Build history of the part. All positions in model axes, mm. A direction names the side the tool comes from. Round coordinates to 2 decimals unless told otherwise and drop trailing zeros. Write each loop counter-clockwise with the first axis right and the second up, starting at its lowest first coordinate (ties: lowest second). Pieces come first, ordered by that corner, then holes. Notation, with made-up numbers: (87.5, 88.5) -> (92.5, 88.5) arc R16 cw to (92.5, 109.5) -> close; hole circle Ø5 at (11.5, 71). An arc over 180 degrees is marked (long way). Answer in a Markdown table with one row per item.
```python
from build123d import *

# Parameters (mm, degrees)
ESBO_O1_R                  = 2.5
RESSALTO_EXTRUS_O1_DEPTH   = 10.6
ESBO_O8_W                  = 21.2
ESBO_O8_H                  = 35
RESSALTO_EXTRUS_O6_DEPTH   = 1.5
RESSALTO_EXTRUS_O2_DEPTH   = 1.5
CORTE_EXTRUS_O1_DEPTH      = 48.855720661
CORTE_EXTRUS_O1_DEPTH_BACK = 48.855720661
ESBO_O3_W                  = 15.2
ESBO_O3_H                  = 37.5
CORTE_EXTRUS_O2_DEPTH      = 48.855720661
CORTE_EXTRUS_O2_DEPTH_BACK = 48.855720661
ESBO_O4_R                  = 0.85
ESBO_O5_W                  = 3
ESBO_O5_H                  = 30
RESSALTO_EXTRUS_O3_DEPTH   = 2.5
RESSALTO_EXTRUS_O4_DEPTH   = 2.5
RESSALTO_EXTRUS_O5_START   = -83.6
ESBO_O7_R                  = 35
RESSALTO_EXTRUS_O5_DEPTH   = 3
NERVURA2_REACH             = 121.79
ESBO_O10_WALL_W            = 274.68518898
ESBO_O10_WALL_H            = 2
ESBO_O11_W                 = 18
ESBO_O11_H                 = 35
RESSALTO_EXTRUS_O7_DEPTH   = 5
ESBO_O12_W                 = 13
ESBO_O12_H                 = 23
CORTE_EXTRUS_O3_DEPTH      = 130.230801453
ESBO_O13_R                 = 0.85
CORTE_EXTRUS_O4_DEPTH      = 130.230801453
ESBO_O14_W                 = 8
ESBO_O14_H                 = 14.1
RESSALTO_EXTRUS_O8_DEPTH   = 5
FILETE1_R                  = 2
NERVURA3_REACH             = 128.994
ESBO_O15_WALL_W            = 11.798728746
ESBO_O15_WALL_H            = 2
ESBO_O16_R                 = 19.8
CORTE_EXTRUS_O5_DEPTH      = 120.428681739
NERVURA4_REACH             = 104.492
ESBO_O17_WALL_W            = 217.06365237
ESBO_O17_WALL_H            = 3


with BuildPart() as part:
    # Esbo_o1 → Ressalto-extrus_o1 (new, symmetric)
    with BuildSketch(Plane(origin=(0, 0, 0), x_dir=(0, 0, -1), z_dir=(1, 0, 0))):
        Circle(ESBO_O1_R)
    extrude(amount=RESSALTO_EXTRUS_O1_DEPTH, both=True)

    # Esbo_o8 → Ressalto-extrus_o6 (add, symmetric)
    with BuildSketch(Plane.XY):
        with Locations((0, -17.5)):
            Rectangle(ESBO_O8_W, ESBO_O8_H)
    extrude(amount=RESSALTO_EXTRUS_O6_DEPTH, both=True)

    # Esbo_o2 → Ressalto-extrus_o2 (add, symmetric)
    with BuildSketch(Plane.XY):
        with BuildLine():
            Line((-10.6, -36), (-10.6, -35))
            Line((-10.6, -35), (-7.6, -35))
            Line((-7.6, -35), (-7.6, -36))
            ThreePointArc((-7.6, -36), (0, -43.6), (7.6, -36))
            Line((7.6, -36), (7.6, -35))
            Line((7.6, -35), (10.6, -35))
            Line((10.6, -35), (10.6, -36))
            ThreePointArc((10.6, -36), (0, -46.6), (-10.6, -36))
        make_face()
    extrude(amount=RESSALTO_EXTRUS_O2_DEPTH, both=True)

    # Esbo_o3 → Corte-extrus_o1 (cut, two sides: drawn at the far end of the back side and taken through both)
    with BuildSketch(Plane.XY.offset(-CORTE_EXTRUS_O1_DEPTH_BACK)):
        with Locations((0, -16.25)):
            Rectangle(ESBO_O3_W, ESBO_O3_H)
    extrude(amount=CORTE_EXTRUS_O1_DEPTH + CORTE_EXTRUS_O1_DEPTH_BACK, mode=Mode.SUBTRACT)

    # Esbo_o4 → Corte-extrus_o2 (cut, two sides: drawn at the far end of the back side and taken through both)
    with BuildSketch(Plane(origin=(0, 0, 0), x_dir=(0, 0, -1), z_dir=(1, 0, 0)).offset(-CORTE_EXTRUS_O2_DEPTH_BACK)):
        Circle(ESBO_O4_R)
    extrude(amount=CORTE_EXTRUS_O2_DEPTH + CORTE_EXTRUS_O2_DEPTH_BACK, mode=Mode.SUBTRACT)

    # Esbo_o5 → Ressalto-extrus_o3 (add, symmetric)
    with BuildSketch(Plane(origin=(0, 0, 0), x_dir=(0, 0, -1), z_dir=(1, 0, 0))):
        with Locations((0, -60.1)):
            Rectangle(ESBO_O5_W, ESBO_O5_H)
    extrude(amount=RESSALTO_EXTRUS_O3_DEPTH, both=True)

    # Esbo_o6 → Ressalto-extrus_o4 (add, symmetric)
    with BuildSketch(Plane(origin=(0, 0, 0), x_dir=(0, 0, -1), z_dir=(1, 0, 0))):
        with BuildLine():
            ThreePointArc((-10, -86.6), (-1.868272016, -83.231727984), (1.5, -75.1))
            ThreePointArc((1.5, -75.1), (0, -73.6), (-1.5, -75.1))
            ThreePointArc((-1.5, -75.1), (-3.98959236, -81.11040764), (-10, -83.6))
            ThreePointArc((-10, -83.6), (-11.5, -85.1), (-10, -86.6))
        make_face()
    extrude(amount=RESSALTO_EXTRUS_O4_DEPTH, both=True)

    # Esbo_o7 → Ressalto-extrus_o5 (add)
    with BuildSketch(Plane(origin=(0, 0, 0), x_dir=(1, 0, 0), z_dir=(0, 1, 0)).offset(RESSALTO_EXTRUS_O5_START)):
        with Locations(Location((0, -40, 0), (0, 0, 270))):
            Circle(ESBO_O7_R)
    extrude(amount=-RESSALTO_EXTRUS_O5_DEPTH)

    # Esbo_o10 wall → Nervura2 (add, up to next)
    with BuildSketch(Plane(origin=(0, -68.6, 8.5), x_dir=(0, -0.906183139995, 0.422885465331), z_dir=(0, -0.422885465331, -0.906183139995)), mode=Mode.PRIVATE) as nervura2_sk1:
        Rectangle(ESBO_O10_WALL_W, ESBO_O10_WALL_H)
    nervura2_tool1 = extrude(nervura2_sk1.sketch, amount=NERVURA2_REACH, mode=Mode.PRIVATE) - part.part
    add(nervura2_tool1.solids().sort_by_distance((0, -68.6, 8.5))[0])



with BuildPart() as body_2:
    # Esbo_o11 → Ressalto-extrus_o7 (new body)
    with BuildSketch(Plane(origin=(19.8, 0, 0), x_dir=(0, 0, -1), z_dir=(1, 0, 0))):
        with Locations((-32.81, -55)):
            Rectangle(ESBO_O11_W, ESBO_O11_H)
    extrude(amount=RESSALTO_EXTRUS_O7_DEPTH)

    # Esbo_o12 → Corte-extrus_o3 (cut, through all)
    with BuildSketch(Plane(origin=(24.8, 0, 0), x_dir=(0, 0, -1), z_dir=(1, 0, 0))):
        with Locations((-32.81, -55)):
            Rectangle(ESBO_O12_W, ESBO_O12_H)
    extrude(amount=-CORTE_EXTRUS_O3_DEPTH, mode=Mode.SUBTRACT)

    # Esbo_o13 → Corte-extrus_o4 (cut, through all)
    with BuildSketch(Plane(origin=(24.8, 0, 0), x_dir=(0, 0, -1), z_dir=(1, 0, 0))):
        with Locations((-32.81, -41)):
            Circle(ESBO_O13_R)
        with Locations((-32.81, -69)):
            Circle(ESBO_O13_R)
    extrude(amount=-CORTE_EXTRUS_O4_DEPTH, mode=Mode.SUBTRACT)


with BuildPart() as part_1:
    add(part.part)

    add(body_2.part)  # Ressalto-extrus_o8 merges body 2
    # Esbo_o14 → Ressalto-extrus_o8 (add)
    with BuildSketch(Plane.ZY.offset(-19.8)):
        with Locations((32.81, -79.55)):
            Rectangle(ESBO_O14_W, ESBO_O14_H)
    extrude(amount=-RESSALTO_EXTRUS_O8_DEPTH)

    # Filete1
    filete1_edges = [part_1.edges().sort_by_distance(p)[0] for p in [
        (22.3, -37.5, 41.81),
        (22.3, -72.5, 41.81),
        (22.3, -72.5, 23.81),
        (22.3, -37.5, 23.81),
    ]]
    fillet(filete1_edges, radius=FILETE1_R)

    # Esbo_o15 wall → Nervura3 (add, up to next)
    with BuildSketch(Plane(origin=(19.8, -81.05, 26.81), x_dir=(0, -0.94077931952, -0.339019574602), z_dir=(0, 0.339019574602, -0.94077931952)), mode=Mode.PRIVATE) as nervura3_sk1:
        with Locations((0, -1)):
            Rectangle(ESBO_O15_WALL_W, ESBO_O15_WALL_H)
    nervura3_tool1 = extrude(nervura3_sk1.sketch, amount=-NERVURA3_REACH, mode=Mode.PRIVATE) - part_1.part
    nervura3 = nervura3_tool1.solids().sort_by_distance((19.8, -81.05, 26.81))[0]
    add(nervura3)

    # Espelhar2: Nervura3 across plane
    add(nervura3.mirror(Plane.XY.offset(32.81)))

    # Esbo_o16 → Corte-extrus_o5 (cut, through all)
    with BuildSketch(Plane(origin=(0, -83.6, 0), x_dir=(1, 0, 0), z_dir=(0, 1, 0))):
        with Locations(Location((0, -40, 0), (0, 0, 270))):
            Circle(ESBO_O16_R)
    extrude(amount=-CORTE_EXTRUS_O5_DEPTH, mode=Mode.SUBTRACT)

    # Esbo_o17 wall → Nervura4 (add, up to next)
    with BuildSketch(Plane(origin=(27.8, -79.55, 32.81), x_dir=(0.595227550626, -0.803557193345, 0), z_dir=(0.803557193345, 0.595227550626, 0)), mode=Mode.PRIVATE) as nervura4_sk1:
        Rectangle(ESBO_O17_WALL_W, ESBO_O17_WALL_H)
    nervura4_tool1 = extrude(nervura4_sk1.sketch, amount=-NERVURA4_REACH, mode=Mode.PRIVATE) - part_1.part
    add(nervura4_tool1.solids().sort_by_distance((27.8, -79.55, 32.81))[0])


solid = part_1.part
```
Q1. Saw through at C-C on x = 18. Write the cut outline in (y, z).
A:
| item | result |
|---|---|
| outline | (-86.6, 9.98) -> (-83.6, 9.98) -> (-83.6, 31.75) -> (-86.6, 31.75) -> close; (-86.6, 48.25) -> (-83.6, 48.25) -> (-83.6, 70.02) -> (-86.6, 70.02) -> close |
Q2. Saw through at A-A on y = -6. Write the cut outline in (x, z), plus the area to 3 significant figures.
A:
| item | result |
|---|---|
| outline | (-10.6, -1.5) -> (-7.6, -1.5) -> (-7.6, 1.5) -> (-10.6, 1.5) -> close; (7.6, -1.5) -> (10.6, -1.5) -> (10.6, 1.5) -> (7.6, 1.5) -> close |
| area | 18.0 mm² |
Q3. Two-plate mould, pull along Y, no slides. Class faces 5 (the flat face through (22, -55, 39.31)), 6 (the flat face through (8, -36, 1.5)), 7 (the cylindrical face through (-0.17, -43.6, 0.02)): released by +Y, released by -Y, zero draft, split by the parting line, or undercut.
A:
| item | result |
|---|---|
| face 5 | undercut |
| face 6 | zero draft |
| face 7 | released by +Y |
Q4. Wall check: line 1 (Z direction, x = -9.6, y = 0); line 2 (X direction, y = -85, z = 40); line 3 (Y direction, x = -27.5, z = 29.5). Give the ranges that are in metal, low to high. Write a range as [from, to].
A:
| item | result |
|---|---|
| line 1 | [-2.5, -0.85], [0.85, 2.5] |
| line 2 | [-35, -19.8], [19.8, 35] |
| line 3 | [-86.6, -83.6] |
Q5. Which spindle directions (+Z, -Z, +X, -X, +Y, -Y) get a long thin tool onto all of the face, cutting with end or side? Do faces 1 (the flat face through (22, -72.5, 38)), 2 (the flat face through (1, -73, 7)), 3 (the flat face through (22, -55, 23.81)), 4 (the flat face through (23, -77, 36.81)). Say none if no direction does.
A:
| item | result |
|---|---|
| face 1 | +Z, +X, -X |
| face 2 | +Z, +X, +Y |
| face 3 | -Z, +X, -X, +Y |
| face 4 | +Z, +X |
Q6. Saw through at B-B on z = 38. Write the cut outline in (x, y).
A:
| item | result |
|---|---|
| outline | (-34.94, -86.6) -> (-19.7, -86.6) -> (-19.7, -83.6) -> (-34.94, -83.6) -> close; (19.7, -86.6) -> (34.94, -86.6) -> (34.94, -83.6) -> (21.8, -83.6) -> (21.8, -78.8) -> (19.8, -78.8) -> (19.8, -83.6) -> (19.7, -83.6) -> close; (19.8, -72.5) -> (24.8, -72.5) -> (24.8, -66.5) -> (19.8, -66.5) -> close; (19.8, -43.5) -> (24.8, -43.5) -> (24.8, -37.5) -> (19.8, -37.5) -> close |
Q7. Drop flat-ended pins along their axis: P1, Ø2.5, axis at x = 21.5, y = -49.5, coming from the -Z side; P2, Ø2, axis at y = 0, z = 0, coming from the -X side; P3, Ø24, axis at x = 0, z = 40, coming from the +Y side; P4, Ø2.5, axis at y = -41, z = 32.81, coming from the +X side. Give the stop position or say it passes through.
A:
| item | result |
|---|---|
| P1 | z = 23.81 |
| P2 | x = -10.6 |
| P3 | through |
| P4 | x = 24.8 |
Q8. Saw through at D-D on y = -57. Write the cut outline in (x, z).
A:
| item | result |
|---|---|
| outline | (-2.5, -1.5) -> (2.5, -1.5) -> (2.5, 1.5) -> (1, 1.5) -> (1, 3.09) -> (-1, 3.09) -> (-1, 1.5) -> (-2.5, 1.5) -> close; (19.8, 23.81) -> (24.8, 23.81) -> (24.8, 26.31) -> (19.8, 26.31) -> close; (19.8, 39.31) -> (24.8, 39.31) -> (24.8, 41.81) -> (19.8, 41.81) -> close |
